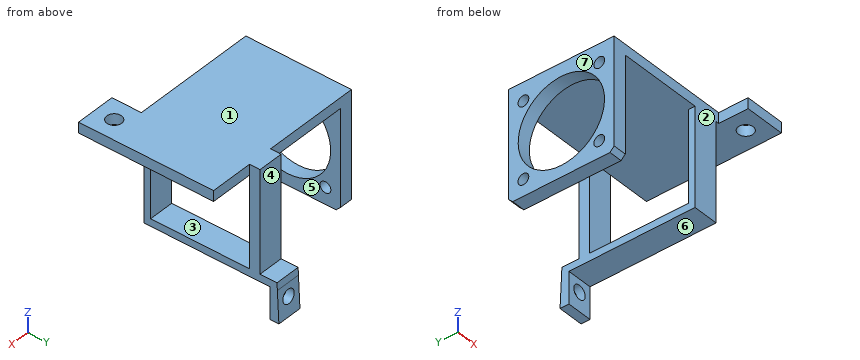
from build123d import *

# Parameters (mm, degrees)
BOSS_EXTRUDE1_DEPTH  = 5
SKETCH2_W            = 6.35
SKETCH2_H            = 50
BOSS_EXTRUDE2_DEPTH  = 52.48
CUT_EXTRUDE1_REACH   = 111.834
SKETCH3_R            = 20.44
SKETCH3_R_2          = 2.555
SKETCH3_W            = 5
SKETCH3_H            = 50
CUT_EXTRUDE2_REACH   = 113.895
SKETCH4_R            = 3.5
CUT_EXTRUDE6_REACH   = 113.895
SKETCH14_W           = 19
SKETCH14_H           = 15.316152196
SKETCH15_W           = 12
SKETCH15_H           = 3.2
BOSS_EXTRUDE7_DEPTH  = 46.5
BOSS_EXTRUDE8_REACH  = 107.356
SKETCH16_W           = 12
SKETCH16_H           = 3.5
SKETCH17_W           = 12
SKETCH17_H           = 3.5
BOSS_EXTRUDE9_DEPTH  = 15
CHAMFER2_SIZE        = 2
SKETCH22_W           = 12
SKETCH22_H           = 15
BOSS_EXTRUDE10_DEPTH = 0.72
CUT_EXTRUDE8_REACH   = 108.012
CUT_EXTRUDE7_REACH   = 125.963
SKETCH18_R           = 3.25
CIRPATTERN2_COUNT    = 2
CIRPATTERN2_ANGLE    = 90
BOSS_EXTRUDE11_REACH = 120.448
SKETCH24_W           = 12
SKETCH24_H           = 5


with BuildPart() as part:
    # Sketch1 → Boss-Extrude1 (new body)
    with BuildSketch(Plane.XY):
        Polygon((0, 0), (0, 50), (46.06, 50), (46.06, 55), (58.06, 55), (58.06, 50), (59.5, 50), (59.5, 64.061014889), (78.5, 64.061014889), (78.5, -13.938985111), (59.5, -13.938985111), (59.5, 0), align=None)
    extrude(amount=BOSS_EXTRUDE1_DEPTH)

    # Sketch2 → Boss-Extrude2 (add)
    with BuildSketch(Plane(origin=(0, 0, 0), x_dir=(-1, 0, 0), z_dir=(0, 0, -1))):
        with Locations((-3.175, 25)):
            Rectangle(SKETCH2_W, SKETCH2_H)
    extrude(amount=BOSS_EXTRUDE2_DEPTH)

    # Sketch3 → Cut-Extrude1 (cut, up to next)
    with BuildSketch(Plane(origin=(6.35, 0, 0), x_dir=(0, 0, -1), z_dir=(1, 0, 0)), mode=Mode.PRIVATE) as cut_extrude1_sk1:
        with Locations((21.66, 25)):
            Circle(SKETCH3_R)
    cut_extrude1_tool1 = extrude(cut_extrude1_sk1.sketch, amount=-CUT_EXTRUDE1_REACH, mode=Mode.PRIVATE) & part.part
    # Sketch3 → Cut-Extrude1 (cut, up to next)
    with BuildSketch(Plane(origin=(6.35, 0, 0), x_dir=(0, 0, -1), z_dir=(1, 0, 0)), mode=Mode.PRIVATE) as cut_extrude1_sk2:
        with Locations((3.695, 42.955)):
            Circle(SKETCH3_R_2)
    cut_extrude1_tool2 = extrude(cut_extrude1_sk2.sketch, amount=-CUT_EXTRUDE1_REACH, mode=Mode.PRIVATE) & part.part
    # Sketch3 → Cut-Extrude1 (cut, up to next)
    with BuildSketch(Plane(origin=(6.35, 0, 0), x_dir=(0, 0, -1), z_dir=(1, 0, 0)), mode=Mode.PRIVATE) as cut_extrude1_sk3:
        with Locations((39.615, 7.045)):
            Circle(SKETCH3_R_2)
    cut_extrude1_tool3 = extrude(cut_extrude1_sk3.sketch, amount=-CUT_EXTRUDE1_REACH, mode=Mode.PRIVATE) & part.part
    # Sketch3 → Cut-Extrude1 (cut, up to next)
    with BuildSketch(Plane(origin=(6.35, 0, 0), x_dir=(0, 0, -1), z_dir=(1, 0, 0)), mode=Mode.PRIVATE) as cut_extrude1_sk4:
        with Locations((49.98, 25)):
            Rectangle(SKETCH3_W, SKETCH3_H)
    cut_extrude1_tool4 = extrude(cut_extrude1_sk4.sketch, amount=-CUT_EXTRUDE1_REACH, mode=Mode.PRIVATE) & part.part
    cut_extrude1_1 = cut_extrude1_tool1.solids().sort_by_distance((6.35, 25, -21.66))[0]
    add(cut_extrude1_1, mode=Mode.SUBTRACT)
    cut_extrude1_2 = cut_extrude1_tool2.solids().sort_by_distance((6.35, 42.955, -3.695))[0]
    add(cut_extrude1_2, mode=Mode.SUBTRACT)
    cut_extrude1_3 = cut_extrude1_tool3.solids().sort_by_distance((6.35, 7.045, -39.615))[0]
    add(cut_extrude1_3, mode=Mode.SUBTRACT)
    cut_extrude1_4 = cut_extrude1_tool4.solids().sort_by_distance((6.35, 25, -49.98))[0]
    add(cut_extrude1_4, mode=Mode.SUBTRACT)
    cut_extrude1 = cut_extrude1_1 + cut_extrude1_2 + cut_extrude1_3 + cut_extrude1_4  # Cut-Extrude1 as one shape, for the pattern or mirror that repeats it

    # Sketch4 → Cut-Extrude2 (cut, up to next)
    with BuildSketch(Plane(origin=(0, 0, 0), x_dir=(-1, 0, 0), z_dir=(0, 0, -1)), mode=Mode.PRIVATE) as cut_extrude2_sk1:
        with Locations((-69, 55.061014889)):
            Circle(SKETCH4_R)
    cut_extrude2_tool1 = extrude(cut_extrude2_sk1.sketch, amount=-CUT_EXTRUDE2_REACH, mode=Mode.PRIVATE) & part.part
    # Sketch4 → Cut-Extrude2 (cut, up to next)
    with BuildSketch(Plane(origin=(0, 0, 0), x_dir=(-1, 0, 0), z_dir=(0, 0, -1)), mode=Mode.PRIVATE) as cut_extrude2_sk2:
        with Locations((-69, -4.938985111)):
            Circle(SKETCH4_R)
    cut_extrude2_tool2 = extrude(cut_extrude2_sk2.sketch, amount=-CUT_EXTRUDE2_REACH, mode=Mode.PRIVATE) & part.part
    add(cut_extrude2_tool1.solids().sort_by_distance((69, 55.061015, 0))[0], mode=Mode.SUBTRACT)
    add(cut_extrude2_tool2.solids().sort_by_distance((69, -4.938985, 0))[0], mode=Mode.SUBTRACT)

    # Sketch14 → Cut-Extrude6 (cut, up to next)
    with BuildSketch(Plane(origin=(0, 0, 0), x_dir=(-1, 0, 0), z_dir=(0, 0, -1)), mode=Mode.PRIVATE) as cut_extrude6_sk1:
        with Locations((-69, 57.658076098)):
            Rectangle(SKETCH14_W, SKETCH14_H)
    cut_extrude6_tool1 = extrude(cut_extrude6_sk1.sketch, amount=-CUT_EXTRUDE6_REACH, mode=Mode.PRIVATE) & part.part
    add(cut_extrude6_tool1.solids().sort_by_distance((69, 57.658076, 0))[0], mode=Mode.SUBTRACT)

    # Sketch15 → Boss-Extrude7 (add)
    with BuildSketch(Plane(origin=(0, 0, 0), x_dir=(-1, 0, 0), z_dir=(0, 0, -1))):
        with Locations((-52.06, 1.6)):
            Rectangle(SKETCH15_W, SKETCH15_H)
    extrude(amount=BOSS_EXTRUDE7_DEPTH)

    # Boss-Extrude8: up to this plane
    boss_extrude8_end = Plane(origin=(166.832994776, 64.085435133, -66.619565524), z_dir=(-1.1416993347548052e-15, 0.9990256874715413, 0.04413247978546202))
    # Sketch16 → Boss-Extrude8 (add, up to the surface)
    with BuildSketch(Plane(origin=(0, 3.2, 0), x_dir=(1, 0, 0), z_dir=(0, 1, 0)), mode=Mode.PRIVATE) as boss_extrude8_sk1:
        with Locations((52.06, 44.75)):
            Rectangle(SKETCH16_W, SKETCH16_H)
    boss_extrude8_tool1 = split(extrude(boss_extrude8_sk1.sketch, amount=BOSS_EXTRUDE8_REACH, mode=Mode.PRIVATE), bisect_by=boss_extrude8_end, keep=Keep.BOTH, mode=Mode.PRIVATE)
    add(boss_extrude8_tool1.solids().sort_by_distance((52.06, 3.2, -44.75))[0])

    # Sketch17 → Boss-Extrude9 (add)
    with BuildSketch(Plane(origin=(0, 0, -46.5), x_dir=(-1, 0, 0), z_dir=(0, 0, -1))):
        with Locations((-52.06, 61.446642853)):
            Rectangle(SKETCH17_W, SKETCH17_H)
    extrude(amount=BOSS_EXTRUDE9_DEPTH)

    # Chamfer2
    chamfer2_edges = [part.edges().sort_by_distance(p)[0] for p in [
        (3.175, 0, -47.48),
        (3.175, 50, -47.48),
    ]]
    chamfer(chamfer2_edges, length=CHAMFER2_SIZE)

    # Sketch22 → Boss-Extrude10 (add)
    with BuildSketch(Plane(origin=(0, 63.196642853, 0), x_dir=(1, 0, 0), z_dir=(0, 1, 0))):
        with Locations((52.06, 54)):
            Rectangle(SKETCH22_W, SKETCH22_H)
    extrude(amount=BOSS_EXTRUDE10_DEPTH)

    # Sketch23 → Cut-Extrude8 (cut, up to next)
    with BuildSketch(Plane(origin=(58.06, 0, 0), x_dir=(0, 0, -1), z_dir=(1, 0, 0)), mode=Mode.PRIVATE) as cut_extrude8_sk1:
        Polygon((46.5, 63.916642853), (46.5, 63.196642853), (61.5, 63.916642853), align=None)
    cut_extrude8_tool1 = extrude(cut_extrude8_sk1.sketch, amount=-CUT_EXTRUDE8_REACH, mode=Mode.PRIVATE) & part.part
    add(cut_extrude8_tool1.solids().sort_by_distance((58.06, 63.676643, -51.5))[0], mode=Mode.SUBTRACT)

    # Cut-Extrude7: up to this plane
    cut_extrude7_end = Plane(origin=(-0.001, 63.196642853, -46.5), z_dir=(-2.1659106514416256e-15, -0.9988499868416298, -0.04794479936839813))
    # Sketch18 → Cut-Extrude7 (cut, up to the surface)
    with BuildSketch(Plane.XZ.offset(-59.696642853), mode=Mode.PRIVATE) as cut_extrude7_sk1:
        with Locations(Location((52.06, -52.57, 0), (0, 0, 270))):
            Circle(SKETCH18_R)
    cut_extrude7_tool1 = split(extrude(cut_extrude7_sk1.sketch, amount=-CUT_EXTRUDE7_REACH, mode=Mode.PRIVATE), bisect_by=cut_extrude7_end, keep=Keep.BOTH, mode=Mode.PRIVATE)
    add(cut_extrude7_tool1.solids().sort_by_distance((52.06, 59.696643, -52.57))[0], mode=Mode.SUBTRACT)

    # CirPattern2: Cut-Extrude1 ×2 about axis
    cirpattern2_axis = Axis((0, 25, -21.66), (-1, 0, 0))
    for i in range(1, CIRPATTERN2_COUNT):
        add(cut_extrude1.rotate(cirpattern2_axis, i * CIRPATTERN2_ANGLE / (CIRPATTERN2_COUNT - 1)), mode=Mode.SUBTRACT)

    # Sketch24 → Boss-Extrude11 (add, up to next)
    with BuildSketch(Plane(origin=(0, 0, 0), x_dir=(-1, 0, 0), z_dir=(0, 0, -1)), mode=Mode.PRIVATE) as boss_extrude11_sk1:
        with Locations((-52.06, 52.5)):
            Rectangle(SKETCH24_W, SKETCH24_H)
    boss_extrude11_tool1 = extrude(boss_extrude11_sk1.sketch, amount=BOSS_EXTRUDE11_REACH, mode=Mode.PRIVATE) - part.part
    add(boss_extrude11_tool1.solids().sort_by_distance((52.06, 52.5, 0))[0])


solid = part.part
Verification items for the finished model (mm, model axes). Face numbers are marked on the shaded views. A direction names the side the tool comes from. Coordinates: 2 decimals unless noted, no trailing zeros. Write each loop counter-clockwise with the first axis right and the second up, starting at its lowest first coordinate (ties: lowest second). Pieces come first, ordered by that corner, then holes. Notation, with made-up numbers: M 22,44 L 62,44 A18 cw 62,48 Z; hole C 80,18 d4. An arc over 180 degrees is marked long. Use a Markdown table: item, result.
Q1. Sectioned sample at D-D, the plane y = 25. Record the boundary of the cut face in (x, z).
Reply:
| item | result |
|---|---|
| outline | M 0,-47.48 L 6.35,-47.48 L 6.35,-42.1 L 0,-42.1 Z; M 0,-1.22 L 6.35,-1.22 L 6.35,0 L 78.5,0 L 78.5,5 L 0,5 Z; M 46.06,-46.5 L 58.06,-46.5 L 58.06,-43 L 46.06,-43 Z |
Q2. Set-up check for the marked faces 1, 2, 3 and 4: record each of +Z, -Z, +X, -X, +Y, -Y from which the full face is reachable in a straight line by a thin tool's end or side.
Reply:
| item | result |
|---|---|
| face 1 | +Z, +X, -X, +Y, -Y |
| face 2 | +Z, -Z, -X, -Y |
| face 3 | +X |
| face 4 | +Z, +X, -X, +Y |
Q3. Sectioned sample at A-A, the plane z = -21.66. Record the boundary of the cut face in (x, y).
Reply:
| item | result |
|---|---|
| outline | M 0,0 L 6.35,0 L 6.35,4.56 L 0,4.56 Z; M 0,45.44 L 6.35,45.44 L 6.35,50 L 0,50 Z; M 46.06,0 L 58.06,0 L 58.06,3.2 L 46.06,3.2 Z; M 46.06,50 L 58.06,50 L 58.06,55 L 46.06,55 Z |
Q4. Draft check along X on the marked faces 5, 6 and 7. Enter one of: +X half, -X half, draft (parallel to the pull), parting line (faces both ways), or undercut.
Reply:
| item | result |
|---|---|
| face 5 | undercut |
| face 6 | draft |
| face 7 | -X half |
Q5. Thickness scan on line 1 (Z direction, x = 49, y = 12); line 2 (Z direction, x = 52, y = 60); line 3 (Y direction, x = 69, z = 1). Record the ranges inside material, lowest first.
Reply:
| item | result |
|---|---|
| line 1 | z = -46.5 to -43, 0 to 5 |
| line 2 | z = -61.5 to -55.82, -49.32 to -43 |
| line 3 | y = -13.94 to -8.44, -1.44 to 50 |
Q6. Sectioned sample at C-C, the plane x = 69. Record the boundary of the cut face in (y, z).
Reply:
| item | result |
|---|---|
| outline | M -13.94,0 L -8.44,0 L -8.44,5 L -13.94,5 Z; M -1.44,0 L 50,0 L 50,5 L -1.44,5 Z |
Q7. Sectioned sample at B-B, the plane x = 52.06. Record the boundary of the cut face in (y, z), plus the area to 3 significant figures.
Reply:
| item | result |
|---|---|
| outline | M 0,-46.5 L 59.7,-46.5 L 59.7,-49.32 L 63.33,-49.32 L 63.2,-46.5 L 63.04,-43 L 55,-43 L 55,5 L 0,5 Z; M 59.7,-61.5 L 63.92,-61.5 L 63.64,-55.82 L 59.7,-55.82 Z; hole M 3.2,-43 L 50,-43 L 50,0 L 3.2,0 Z |
| area | 882 mm² |
Q8. Go/stop test with flat-tipped pins: P1, Ø3, axis at y = 55.5, z = -35, coming from the -X side; P2, Ø23.5, axis at y = 27.5, z = -13, coming from the +X side; P3, Ø4, axis at x = 71.5, z = 2, coming from the +Y side; P4, Ø8, axis at y = 9.5, z = -25, coming from the -X side. Record where each tip stops, or that it passes through.
Reply:
| item | result |
|---|---|
| P1 | stops at x = 46.06 |
| P2 | stops at x = 6.35 |
| P3 | stops at y = 50 |
| P4 | passes through |
